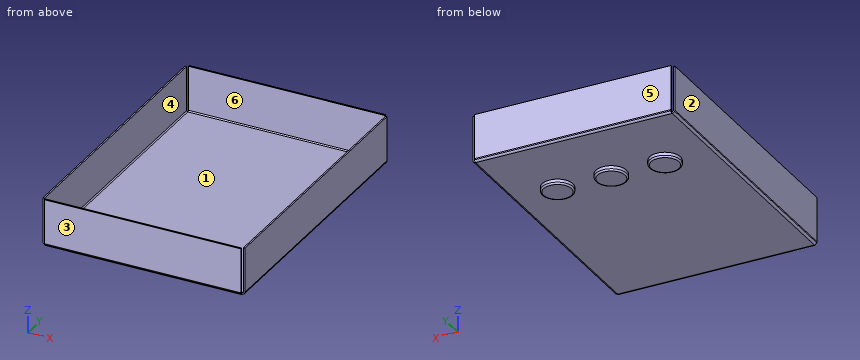
```python
from build123d import *

# Parameters (mm, degrees)
BASE_FLANGE1_DEPTH         = 1
SKETCHED_START             = 31
SKETCHED_BEND1_DEPTH       = 178
SKETCHED_BEND1_2_DEPTH     = 128
SKETCHED_BEND1_3_DEPTH     = 178
SKETCHED_BEND1_4_OUTLINE_W = 128
SKETCHED_BEND1_4_OUTLINE_H = 1
SKETCHED_BEND1_4_DEPTH     = 29.234623369
SKETCHED_START_2           = 210.765376631
SKETCHED_BEND1_5_OUTLINE_W = 128
SKETCHED_BEND1_5_OUTLINE_H = 1
SKETCHED_BEND1_5_DEPTH     = 29.234623369
SKETCHED_BEND1_6_DEPTH     = 128
SKETCHED_BEND1_7_OUTLINE_W = 178
SKETCHED_BEND1_7_OUTLINE_H = 1
SKETCHED_BEND1_7_DEPTH     = 29.234623369
SKETCHED_START_3           = 160.765376631
SKETCHED_BEND1_8_OUTLINE_W = 178
SKETCHED_BEND1_8_OUTLINE_H = 1
SKETCHED_BEND1_8_DEPTH     = 29.234623369
SKETCH7_R                  = 10
BOSS_EXTRUDE1_DEPTH        = 3
FILLET1_R                  = 1


# Read off the part's stored shape, not the designer's step: Sketched Bend1
# Sheet-metal steps are written as plain solids
with BuildPart() as part:
    # Sketch1 → Base-Flange1 (new body)
    with BuildSketch(Plane.XY):
        Polygon((0, 209), (31, 209), (31, 240), (159, 240), (159, 209), (190, 209), (190, 31), (159, 31), (159, 0), (31, 0), (31, 31), (0, 31), align=None)
    extrude(amount=-BASE_FLANGE1_DEPTH)

    # Sketched Bend1 outline → Sketched Bend1 (add)
    with BuildSketch(Plane(origin=(0, 0, 0), x_dir=(1, 0, 0), z_dir=(0, 1, 0)).offset(SKETCHED_START)):
        with BuildLine():
            Line((29.234623369, -0.7366), (29.234623369, -29.765376631))
            Line((29.234623369, -29.765376631), (30.234623369, -29.765376631))
            Line((30.234623369, -29.765376631), (30.234623369, -0.7366))
            ThreePointArc((30.234623369, -0.7366), (30.450368514, -0.215745145), (30.971223369, 0))
            Line((30.971223369, 0), (29.398582279, 0))
            ThreePointArc((29.398582279, 0), (29.276108612, -0.359286442), (29.234623369, -0.7366))
        make_face()
        with BuildLine():
            Line((160.601417721, 0), (159.028776631, 0))
            ThreePointArc((159.028776631, 0), (159.549631486, -0.215745145), (159.765376631, -0.7366))
            Line((159.765376631, -0.7366), (159.765376631, -29.765376631))
            Line((159.765376631, -29.765376631), (160.765376631, -29.765376631))
            Line((160.765376631, -29.765376631), (160.765376631, -0.7366))
            ThreePointArc((160.765376631, -0.7366), (160.723891388, -0.359286442), (160.601417721, 0))
        make_face()
    extrude(amount=SKETCHED_BEND1_DEPTH)

    # Sketched Bend1 2 outline → Sketched Bend1 2 (add)
    with BuildSketch(Plane.YZ.offset(SKETCHED_START)):
        with BuildLine():
            Line((209.028776631, 0), (210.601417721, 0))
            ThreePointArc((210.601417721, 0), (210.723891388, 0.359286442), (210.765376631, 0.7366))
            Line((210.765376631, 0.7366), (210.765376631, 29.765376631))
            Line((210.765376631, 29.765376631), (209.765376631, 29.765376631))
            Line((209.765376631, 29.765376631), (209.765376631, 0.7366))
            ThreePointArc((209.765376631, 0.7366), (209.549631486, 0.215745145), (209.028776631, 0))
        make_face()
        with BuildLine():
            ThreePointArc((29.234623369, 0.7366), (29.276108612, 0.359286442), (29.398582279, 0))
            Line((29.398582279, 0), (30.971223369, 0))
            ThreePointArc((30.971223369, 0), (30.450368514, 0.215745145), (30.234623369, 0.7366))
            Line((30.234623369, 0.7366), (30.234623369, 29.765376631))
            Line((30.234623369, 29.765376631), (29.234623369, 29.765376631))
            Line((29.234623369, 29.765376631), (29.234623369, 0.7366))
        make_face()
    extrude(amount=SKETCHED_BEND1_2_DEPTH)

    # Sketched Bend1 3 outline → Sketched Bend1 3 (cut)
    with BuildSketch(Plane(origin=(0, 0, 0), x_dir=(1, 0, 0), z_dir=(0, 1, 0)).offset(SKETCHED_START)):
        with BuildLine():
            Line((0, 0), (29.398582279, 0))
            ThreePointArc((29.398582279, 0), (30.039397205, 0.728828115), (30.971223369, 1))
            Line((30.971223369, 1), (0, 1))
            Line((0, 1), (0, 0))
        make_face()
        with BuildLine():
            Line((190, 1), (159.028776631, 1))
            ThreePointArc((159.028776631, 1), (159.960602795, 0.728828115), (160.601417721, 0))
            Line((160.601417721, 0), (190, 0))
            Line((190, 0), (190, 1))
        make_face()
    extrude(amount=SKETCHED_BEND1_3_DEPTH, mode=Mode.SUBTRACT)

    # Sketched Bend1 4 outline → Sketched Bend1 4 (cut)
    with BuildSketch(Plane(origin=(0, 0, 0), x_dir=(1, 0, 0), z_dir=(0, 1, 0))):
        with Locations((95, 0.5)):
            Rectangle(SKETCHED_BEND1_4_OUTLINE_W, SKETCHED_BEND1_4_OUTLINE_H)
    extrude(amount=SKETCHED_BEND1_4_DEPTH, mode=Mode.SUBTRACT)

    # Sketched Bend1 5 outline → Sketched Bend1 5 (cut)
    with BuildSketch(Plane(origin=(0, 0, 0), x_dir=(1, 0, 0), z_dir=(0, 1, 0)).offset(SKETCHED_START_2)):
        with Locations((95, 0.5)):
            Rectangle(SKETCHED_BEND1_5_OUTLINE_W, SKETCHED_BEND1_5_OUTLINE_H)
    extrude(amount=SKETCHED_BEND1_5_DEPTH, mode=Mode.SUBTRACT)

    # Sketched Bend1 6 outline → Sketched Bend1 6 (cut)
    with BuildSketch(Plane.YZ.offset(SKETCHED_START)):
        with BuildLine():
            ThreePointArc((210.601417721, 0), (209.960602795, -0.728828115), (209.028776631, -1))
            Line((209.028776631, -1), (240, -1))
            Line((240, -1), (240, 0))
            Line((240, 0), (210.601417721, 0))
        make_face()
        with BuildLine():
            Line((0, -1), (30.971223369, -1))
            ThreePointArc((30.971223369, -1), (30.039397205, -0.728828115), (29.398582279, 0))
            Line((29.398582279, 0), (0, 0))
            Line((0, 0), (0, -1))
        make_face()
    extrude(amount=SKETCHED_BEND1_6_DEPTH, mode=Mode.SUBTRACT)

    # Sketched Bend1 7 outline → Sketched Bend1 7 (cut)
    with BuildSketch(Plane.YZ):
        with Locations((120, -0.5)):
            Rectangle(SKETCHED_BEND1_7_OUTLINE_W, SKETCHED_BEND1_7_OUTLINE_H)
    extrude(amount=SKETCHED_BEND1_7_DEPTH, mode=Mode.SUBTRACT)

    # Sketched Bend1 8 outline → Sketched Bend1 8 (cut)
    with BuildSketch(Plane.YZ.offset(SKETCHED_START_3)):
        with Locations((120, -0.5)):
            Rectangle(SKETCHED_BEND1_8_OUTLINE_W, SKETCHED_BEND1_8_OUTLINE_H)
    extrude(amount=SKETCHED_BEND1_8_DEPTH, mode=Mode.SUBTRACT)

    # Sketch7 → Boss-Extrude1 (add)
    with BuildSketch(Plane(origin=(0, 0, -1), x_dir=(-1, 0, 0), z_dir=(0, 0, -1))):
        with Locations((-130.765376631, 160.765376631)):
            Circle(SKETCH7_R)
        with Locations((-95.765376631, 160.765376631)):
            Circle(SKETCH7_R)
        with Locations((-60.765376631, 160.765376631)):
            Circle(SKETCH7_R)
    extrude(amount=BOSS_EXTRUDE1_DEPTH)

    # Fillet1
    fillet1_edges = [part.edges().sort_by_distance(p)[0] for p in [
        (140.765376631, 160.765376631, -4),
        (105.765376631, 160.765376631, -4),
        (70.765376631, 160.765376631, -4),
    ]]
    fillet(fillet1_edges, radius=FILLET1_R)


solid = part.part
```
The model under review builds one solid part; all positions refer to its coordinate system, in mm. Face numbers are marked on the shaded views. A direction names the side the tool comes from. Round coordinates to 2 decimals unless told otherwise and drop trailing zeros. Order: outer loops, then holes, each group sorted by start corner. A loop starts at its lowest first (then second) coordinate and runs counter-clockwise, first axis right, second up. Notation, with made-up numbers: (-1, -17.75) - (42, -17.75) arc R19 ccw to (42, 5.25) - close; hole circle Ø8 at (25.5, 23.5). An arc over 180 degrees is marked (long way). Answer in a Markdown table with one row per item.
(1) Machinability: for the marked faces 4, 5 and 6, which of the approach directions +Z, -Z, +X, -X, +Y, -Y give a long, thin tool a straight path to every point of the face, cutting with its end or side? Answer none if there is none.
Result set:
| item | result |
|---|---|
| face 4 | +Z, +Y, -Y |
| face 5 | +Z, -Z, +X, -X, +Y |
| face 6 | +Z, +X, -X |
(2) Take a section at C-C on y = 52. Write out the cut boundary in (x, z).
Result set:
| item | result |
|---|---|
| outline | (29.23, 0.74) arc R1.74 ccw to (30.97, -1) - (159.03, -1) arc R1.74 ccw to (160.77, 0.74) - (160.77, 29.77) - (159.77, 29.77) - (159.77, 0.74) arc R0.74 cw to (159.03, 0) - (30.97, 0) arc R0.74 cw to (30.23, 0.74) - (30.23, 29.77) - (29.23, 29.77) - close |
(3) Mouldability with a two-part tool opening along Y and no side actions: class the marked faces 1, 2 and 3 as released by +Y, released by -Y, zero draft, split by the parting line, or undercut.
Result set:
| item | result |
|---|---|
| face 1 | undercut |
| face 2 | zero draft |
| face 3 | released by -Y |
(4) Take a section at B-B on x = 151.5. Write out the cut boundary in (y, z).
Result set:
| item | result |
|---|---|
| outline | (29.23, 0.74) arc R1.74 ccw to (30.97, -1) - (209.03, -1) arc R1.74 ccw to (210.77, 0.74) - (210.77, 29.77) - (209.77, 29.77) - (209.77, 0.74) arc R0.74 cw to (209.03, 0) - (30.97, 0) arc R0.74 cw to (30.23, 0.74) - (30.23, 29.77) - (29.23, 29.77) - close |
(5) Take a section at A-A on z = 8.5. Write out the cut boundary in (x, y).
Result set:
| item | result |
|---|---|
| outline | (29.23, 31) - (30.23, 31) - (30.23, 209) - (29.23, 209) - close; (31, 29.23) - (159, 29.23) - (159, 30.23) - (31, 30.23) - close; (31, 209.77) - (159, 209.77) - (159, 210.77) - (31, 210.77) - close; (159.77, 31) - (160.77, 31) - (160.77, 209) - (159.77, 209) - close |
(6) Clearance check with flat-ended pins moving along their axes: P1, Ø0.5, axis at x = 160, z = 18.5, coming from the -Y side; P2, Ø1.9, axis at y = 30, z = 12, coming from the -X side; P3, Ø8, axis at x = 70.5, y = 48.5, coming from the -Z side. State where each tip first meets the part, or that it passes through.
Result set:
| item | result |
|---|---|
| P1 | stops at y = 31 |
| P2 | stops at x = 31 |
| P3 | stops at z = -1 |
(7) For line 1 (X direction, y = 58, z = 0.5); line 2 (Y direction, x = 147, z = 18.5); line 3 (X direction, y = 126.5, z = 16), list the stretches that pass through material, from the lowest coordinate up. Write a range as from..to.
Result set:
| item | result |
|---|---|
| line 1 | x = 29.25..30.27, 159.73..160.75 |
| line 2 | y = 29.23..30.23, 209.77..210.77 |
| line 3 | x = 29.23..30.23, 159.77..160.77 |
